Geometry: final body of the model. Coordinates: model frame, mm. A direction names the side the tool comes from. Coordinates: 2 decimals unless noted, no trailing zeros. Loops run counter-clockwise (first coordinate to the right, second up) from the corner with the lowest first, then second, coordinate; pieces in that order, holes last. Notation, with made-up numbers: (42.5, -14) -> (77.5, -14) arc R19 ccw to (77.5, 16) -> close; hole circle Ø7 at (86.5, 87). An arc over 180 degrees is marked (long way). One line per item, written item: value. Start each with the question number.
Item 1: Section query C-C on y = 35. Return loops of the section in (x, z), then the cut area to 3 significant figures.
Item 2: Contact query for flat-ended pins moving along their axis: pin 1 Ø4 at (x, z) = (0, -13.5) entering from -Y; pin 2 Ø18.5 at (x, y) = (-15, -13) entering from +Z; pin 3 Ø4 at (x, y) = (-27.5, 10.5) entering from -Z. Output: stop coordinate, or through.
Item 3: Ray query, probe 1 along Y at (x, z) = (-1, -2); probe 2 along X at (y, z) = (-31, -14.25); probe 3 along X at (y, z) = (1, -6.75). Return the intervals inside material, ascending. Write a range as from..to.
Item 4: Section query D-D on z = -13.5. Give the number of separate pieces and of enclosed holes in the cut face, then the cut area to 3 significant figures.
Item 5: Section query B-B on x = 0. Return loops of the section in (y, z).
Item 6: Section query A-A on y = 0. Return loops of the section in (x, z), then the cut area to 3 significant figures.
Item 7: Set-up query: faces 3 (the cylindrical face through (-4.036, 30.736, -2.958)), 4 (the flat face through (9, -24, -9.5)), 5 (the cylindrical face through (19.885, 29.56, -7.605)). Return all of +Z, -Z, +X, -X, +Y, -Y with unobstructed straight access to the full face (end or side cutting, diameter ignored); none if empty.
Item 8: Mould query, pull axis X, two halves, no side actions, for faces 1 (the flat face through (-25.1, -18.5, 0)), 2 (the cylindrical face through (-8.985, -22.542, -12.288)). Classes: +X half, -X half, draft (parallel to the pull), parting line (faces both ways), or undercut.
from build123d import *

# Parameters (mm, degrees)
F0_R             = 42
F0_R_2           = 23
F1_DEPTH         = 15
F2_R             = 31
F2_R_2           = 23
F3_DEPTH         = 6
F4_R             = 3
F5_DEPTH         = 15.001
F7_D             = 5
F7_COPIES_COUNT  = 6
F8_R             = 2
F9_DEPTH         = 15.001
F11_D            = 4.5
F11_CBORE_D      = 7.5
F11_CBORE_DEPTH  = 5.5
F11_COPIES_COUNT = 8


# Not quite as in the source:
# - a pattern or mirror of a feature is missing from the dataset's text; its kind, count and spacing are read off the source's solid


with BuildPart() as f1:
    # F0 (on Top) → F1 (new body)
    with BuildSketch(Plane.XY):
        Circle(F0_R)
        Circle(F0_R_2, mode=Mode.SUBTRACT)
    extrude(amount=-F1_DEPTH)

    # F2 (on face) → F3 (cut)
    with BuildSketch(Plane.XY):
        Circle(F2_R)
        Circle(F2_R_2, mode=Mode.SUBTRACT)
    extrude(amount=-F3_DEPTH, mode=Mode.SUBTRACT)

    # F4 (on face) → F5 (cut, through all)
    with BuildSketch(Plane.XY):
        with Locations((0, -35)):
            Circle(F4_R)
        with Locations((0, 35)):
            Circle(F4_R)
    extrude(amount=-F5_DEPTH, mode=Mode.SUBTRACT)

    # F7 (through all)
    with Locations(Plane.XY):
        with Locations((-17.5, 30.3108891325)):
            f7 = Hole(F7_D / 2)

    # F7_copies: F7 ×6 about axis
    f7_copies_axis = Axis((0, 0, 0), (0, 0, 1))
    for i in range(1, F7_COPIES_COUNT):
        add(f7.rotate(f7_copies_axis, i * 360 / F7_COPIES_COUNT), mode=Mode.SUBTRACT)

    # F8 (on face) → F9 (cut, through all)
    with BuildSketch(Plane(origin=(0, 0, -15), x_dir=(1, 0, 0), z_dir=(0, 0, -1))):
        with Locations((0, -28)):
            Circle(F8_R)
    extrude(amount=-F9_DEPTH, mode=Mode.SUBTRACT)

    # F11 (through all)
    with Locations(Plane(origin=(0, 0, -15), x_dir=(1, 0, 0), z_dir=(0, 0, -1))):
        with Locations((-10.7151361062, 25.8686269103)):
            f11 = CounterBoreHole(F11_D / 2, F11_CBORE_D / 2, F11_CBORE_DEPTH)

    # F11_copies: F11 ×8 about axis
    f11_copies_axis = Axis((0, 0, 0), (0, 0, 1))
    for i in range(1, F11_COPIES_COUNT):
        add(f11.rotate(f11_copies_axis, i * 360 / F11_COPIES_COUNT), mode=Mode.SUBTRACT)


solid = f1.part
Reply:
1. outline: (-23.22, -15) -> (-3, -15) -> (-3, 0) -> (-23.22, 0) -> close; (3, -15) -> (23.22, -15) -> (23.22, 0) -> (3, 0) -> close
1. area: 606 mm²
2. pin 1: stops at y = -42
2. pin 2: stops at z = -6
2. pin 3: stops at z = -9.5
3. probe 1: y = -41.99..-37.83, -32.17..-30.98, 30.98..32.17, 37.83..41.99
3. probe 2: x = -28.34..-19.9, -15.1..15.1, 19.9..28.34
3. probe 3: x = -41.99..-37.29, -32.71..-22.98, 22.98..32.71, 37.29..41.99
4. separate pieces: 1
4. enclosed holes: 18
4. area: 3,340 mm²
5. outline: (-42, -15) -> (-38, -15) -> (-38, 0) -> (-42, 0) -> close; (-32, -15) -> (-23, -15) -> (-23, -6) -> (-31, -6) -> (-31, 0) -> (-32, 0) -> close; (23, -15) -> (26, -15) -> (26, -6) -> (23, -6) -> close; (30, -15) -> (32, -15) -> (32, 0) -> (31, 0) -> (31, -6) -> (30, -6) -> close; (38, -15) -> (42, -15) -> (42, 0) -> (38, 0) -> close
6. outline: (-42, -15) -> (-37.5, -15) -> (-37.5, 0) -> (-42, 0) -> close; (-32.5, -15) -> (-23, -15) -> (-23, -6) -> (-31, -6) -> (-31, 0) -> (-32.5, 0) -> close; (23, -15) -> (32.5, -15) -> (32.5, 0) -> (31, 0) -> (31, -6) -> (23, -6) -> close; (37.5, -15) -> (42, -15) -> (42, 0) -> (37.5, 0) -> close
6. area: 324 mm²
7. face 3: +Z
7. face 4: -Z
7. face 5: +Z, -Z
8. face 1: draft
8. face 2: undercut
